```python
from build123d import *

# Parameters (mm, degrees)
BOSS_EXTRUDE1_DEPTH     = 20
FILLET1_R               = 1
SKETCH2_R               = 4
CUT_EXTRUDE1_DEPTH      = 15
SKETCH3_R               = 5
CUT_EXTRUDE2_DEPTH      = 15
CUT_EXTRUDE3_DEPTH      = 46.069390988
CUT_EXTRUDE3_DEPTH_BACK = 46.069390988
SKETCH4_R               = 4.1
SKETCH4_R_2             = 4


with BuildPart() as part:
    # Sketch1 → Boss-Extrude1 (new body)
    with BuildSketch(Plane(origin=(0, 0, 0), x_dir=(1, 0, 0), z_dir=(0, 1, 0))):
        with BuildLine():
            Line((-9.583148475, 20.357142857), (-19.16629695, -11.785714286))
            ThreePointArc((-19.16629695, -11.785714286), (0, -37.5), (19.16629695, -11.785714286))
            Line((19.16629695, -11.785714286), (9.583148475, 20.357142857))
            ThreePointArc((9.583148475, 20.357142857), (0, 27.5), (-9.583148475, 20.357142857))
        make_face()
    extrude(amount=BOSS_EXTRUDE1_DEPTH)

    # Fillet1
    fillet1_edges = [part.edges().sort_by_distance(p)[0] for p in [
        (0, 20, -27.5),
        (-14.374722712, 20, -4.285714286),
        (0, 20, 37.5),
        (-14.374722712, 0, -4.285714286),
        (0, 0, -27.5),
        (14.374722712, 0, -4.285714286),
        (0, 0, 37.5),
        (14.374722712, 20, -4.285714286),
    ]]
    fillet(fillet1_edges, radius=FILLET1_R)

    # Sketch2 → Cut-Extrude1 (cut)
    with BuildSketch(Plane(origin=(0, 0, 0), x_dir=(1, 0, 0), z_dir=(0, 1, 0))):
        with Locations(Location((0, 15, 0), (0, 0, 270))):
            Circle(SKETCH2_R)
    extrude(amount=CUT_EXTRUDE1_DEPTH, mode=Mode.SUBTRACT)

    # Sketch3 → Cut-Extrude2 (cut)
    with BuildSketch(Plane.XZ.offset(-20)):
        with Locations(Location((0, 0, 0), (0, 0, 270))):
            Circle(SKETCH3_R)
    extrude(amount=CUT_EXTRUDE2_DEPTH, mode=Mode.SUBTRACT)

    # Sketch4 → Cut-Extrude3 (cut, two sides: drawn at the far end of the back side and taken through both)
    with BuildSketch(Plane(origin=(0, 5, 0), x_dir=(-1, 0, 0), z_dir=(0, 1, 0)).offset(-CUT_EXTRUDE3_DEPTH_BACK)):
        with Locations(Location((0, 0, 0), (0, 0, 90))):
            Circle(SKETCH4_R)
        with Locations(Location((0, -15, 0), (0, 0, 90))):
            Circle(SKETCH4_R_2)
    extrude(amount=CUT_EXTRUDE3_DEPTH + CUT_EXTRUDE3_DEPTH_BACK, mode=Mode.SUBTRACT)


solid = part.part
```
Model file for the job. Use its own axes, mm. A direction names the side the tool comes from. Give positions to 0.01 mm unless a question says otherwise; leave off trailing zeros. Order: outer loops, then holes, each group sorted by start corner. A loop starts at its lowest first (then second) coordinate and runs counter-clockwise, first axis right, second up.
1) 3-axis set-ups, long thin cutter, end or side, ignore diameter. For faces 4 (the flat face through (0, 20, 12)), 5 (the flat face through (2, 5, 4)): which of +Z, -Z, +X, -X, +Y, -Y reach the whole face in a straight line?
2) Saw through at A-A, the plane x = 0. Write the cut outline in (y, z).
3) Wall check: probe 1 along Z at (x, y) = (-2.5, 11.5); probe 2 along Z at (x, y) = (3, 3.5); probe 3 along X at (y, z) = (15.25, -15). Give the ranges that are in metal, low to high.
4) Pin check, flat tips, straight feed: pin 1 (5 mm diameter, centred on y = 9, z = -20, fed in from -X) (3 decimals); pin 2 (2 mm diameter, centred on y = 7.5, z = 27.5, fed in from +X); pin 3 (9 mm diameter, centred on x = 0, z = 0, fed in from +Y). Stop position of each tip, or through.
5) Mould opens along Z. For faces 1 (the cylindrical face through (0.2, 9.9, -27.5)), 2 (the cylindrical face through (-0.521, 9.874, 37.493)), 3 (the cylindrical face through (-4.88, 12.6, 1.08)) say: +Z half, -Z half, draft (parallel to the pull), parting line (faces both ways), or undercut.
6) Saw through at B-B, the plane y = 16. Write the cut outline in (x, z).
Computed:
1. face 4: +Z, -Z, +X, -X, +Y
1. face 5: +Y
2. outline: (0, -26.5) arc R1 ccw to (1, -27.5) - (19, -27.5) arc R1 ccw to (20, -26.5) - (20, -19) - (0, -19) - close; (0, -11) - (20, -11) - (20, -5) - (5, -5) - (5, -4.1) - (0, -4.1) - close; (0, 4.1) - (5, 4.1) - (5, 5) - (20, 5) - (20, 36.5) arc R1 ccw to (19, 37.5) - (1, 37.5) arc R1 ccw to (0, 36.5) - close
3. probe 1: z = -27.18 to -18.12, -11.88 to -4.33, 4.33 to 37.34
3. probe 2: z = -27.04 to -17.65, -12.35 to -2.79, 2.79 to 37.27
3. probe 3: x = -11.18 to -4, 4 to 11.18
4. pin 1: stops at x = -10.435
4. pin 2: stops at x = 17.86
4. pin 3: stops at y = 5
5. face 1: -Z half
5. face 2: parting line
5. face 3: undercut
6. outline: (-19.17, 11.79) - (-9.58, -20.36) arc R10 ccw to (9.58, -20.36) - (19.17, 11.79) arc R20 ccw (long way) to start; hole circle Ø10 at (0, 0); hole circle Ø8 at (0, -15)
